Read the model definition and answer for the solid it produces. Units are mm, in the model's axes. Face numbers are marked on the shaded views. A direction names the side the tool comes from. Coordinates: 2 decimals unless noted, no trailing zeros. Write each loop counter-clockwise with the first axis right and the second up, starting at its lowest first coordinate (ties: lowest second). Pieces come first, ordered by that corner, then holes.
Item 1: Section B-B (x = 1) is taken. Give the vertices of the cut face in (y, z).
Item 2: A tool of negligible diameter and unlimited length cuts with its end or side. For the marked faces 1, 2 and 3, from which of +Z, -Z, +X, -X, +Y, -Y can it reach the whole face along a straight path? Write none if from no direction.
Item 3: Section A-A (y = -25) is taken. Give the vertices of the cut face in (x, z).
Item 4: Straight lines are drawn through the part: probe 1 along Z at (x, y) = (3.5, -25); probe 2 along X at (y, z) = (-35, 14.5); probe 3 along Y at (x, z) = (1.25, 13.5). For each, find the intervals that lie inside material, in ascending order.
Item 5: Determine the mould class of the marked faces 4, 5 and 6 for opening direction Z: released by +Z, released by -Z, zero draft, split by the parting line, or undercut.
Item 6: Section C-C (z = 13.9) is taken. Give the vertices of the cut face in (x, y), then the cut area to 3 significant figures.
Item 7: Section D-D (y = -5) is taken. Give the vertices of the cut face in (x, z).
Item 8: Each of these flat-tipped pins is pushed along its axis until it touches: P1, Ø5, axis at x = 7, y = -43.5, coming from the +Z side; P2, Ø1, axis at x = 4, y = -11.5, coming from the +Z side; P3, Ø8, axis at y = -36.5, z = 11.5, coming from the +X side. Where does it stop, or does it pass through?
from build123d import *

# Parameters (mm, degrees)
SKETCH_W        = 14
SKETCH_H        = 19.8
PAD_DEPTH       = 50
POCKET_DEPTH    = 50.001
SKETCH002_R     = 2.7
POCKET001_DEPTH = 10.001
POCKET002_DEPTH = 10


with BuildPart() as part:
    # Sketch → Pad (new body)
    with BuildSketch(Plane.XZ):
        with Locations((7, 9.9)):
            Rectangle(SKETCH_W, SKETCH_H)
    extrude(amount=PAD_DEPTH)

    # Sketch001 (on Face5 of Pad) → Pocket (cut, through all)
    with BuildSketch(Plane(origin=(0, 0, 0), x_dir=(1, 0, 0), z_dir=(0, 1, 0))):
        Polygon((10, -19.8), (10, -8), (12.143594, 0), (14, 0), (14, -19.8), align=None)
    extrude(amount=-POCKET_DEPTH, mode=Mode.SUBTRACT)

    # Sketch002 (on Face6 of Pocket) → Pocket001 (cut, through all)
    with BuildSketch(Plane(origin=(10, 0, 0), x_dir=(0, 0, 1), z_dir=(1, 0, 0))):
        with Locations((13.9, 25)):
            Circle(SKETCH002_R)
    extrude(amount=-POCKET001_DEPTH, mode=Mode.SUBTRACT)

    # Sketch003 (on Face7 of Pocket001) → Pocket002 (cut)
    with BuildSketch(Plane(origin=(10, 0, 0), x_dir=(0, 0, 1), z_dir=(1, 0, 0))):
        Polygon((7.9, 39.9), (19.8, 32.4), (19.8, 50), (7.9, 50), align=None)
        Polygon((7.9, 0), (19.8, 0), (19.8, 17.6), (7.9, 10.1), align=None)
    extrude(amount=-POCKET002_DEPTH, mode=Mode.SUBTRACT)


solid = part.part
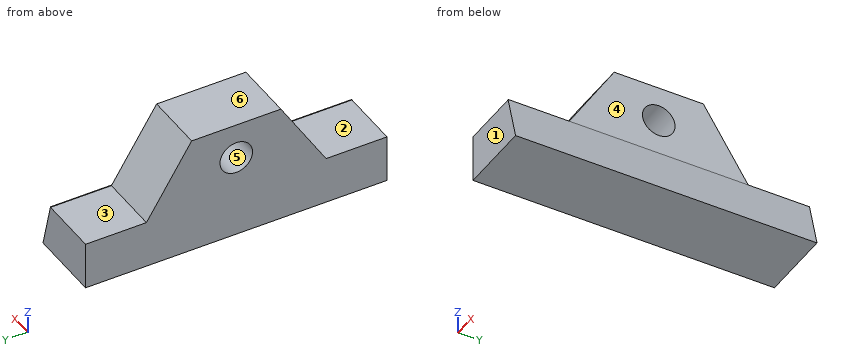
Established:
1. outline: (-50, 0) - (0, 0) - (0, 7.9) - (-10.1, 7.9) - (-17.6, 19.8) - (-32.4, 19.8) - (-39.9, 7.9) - (-50, 7.9) - close; hole circle Ø5.4 at (-25, 13.9)
2. face 1: +Z, -Z, +X, -X, -Y
2. face 2: +Z, -X, -Y
2. face 3: +Z, -X, +Y
3. outline: (0, 0) - (12.14, 0) - (10, 8) - (10, 11.2) - (0, 11.2) - close; (0, 16.6) - (10, 16.6) - (10, 19.8) - (0, 19.8) - close
4. probe 1: z = 0 to 11.2, 16.6 to 19.8
4. probe 2: x = 0 to 10
4. probe 3: y = -36.37 to -27.67, -22.33 to -13.63
5. face 4: zero draft
5. face 5: undercut
5. face 6: released by +Z
6. outline: (0, -36.12) - (10, -36.12) - (10, -27.7) - (0, -27.7) - close; (0, -22.3) - (10, -22.3) - (10, -13.88) - (0, -13.88) - close
6. area: 168 mm2
7. outline: (0, 0) - (12.14, 0) - (10, 8) - (10, 7.9) - (0, 7.9) - close
8. P1: stops at z = 7.9
8. P2: stops at z = 10.91
8. P3: stops at x = 10.13
